Part model, mm, in its own coordinate system. A direction names the side the tool comes from. Round coordinates to 2 decimals unless told otherwise and drop trailing zeros. Loops run counter-clockwise (first coordinate to the right, second up) from the corner with the lowest first, then second, coordinate; pieces in that order, holes last.
from build123d import *

# Parameters (mm, degrees)
SKETCH1_W           = 84
SKETCH1_H           = 300
SKETCH1_W_2         = 54
SKETCH1_H_2         = 80
BOSS_EXTRUDE1_DEPTH = 6
SKETCH2_R           = 1
CUT_EXTRUDE1_DEPTH  = 10
SKETCH4_R           = 1
CUT_EXTRUDE3_DEPTH  = 10
SKETCH5_R           = 1
CUT_EXTRUDE4_DEPTH  = 10


with BuildPart() as part:
    # Sketch1 → Boss-Extrude1 (new body)
    with BuildSketch(Plane.XY):
        Rectangle(SKETCH1_W, SKETCH1_H)
        with Locations((0, 95)):
            Rectangle(SKETCH1_W_2, SKETCH1_H_2, mode=Mode.SUBTRACT)
        with Locations((0, -95)):
            Rectangle(SKETCH1_W_2, SKETCH1_H_2, mode=Mode.SUBTRACT)
        Rectangle(SKETCH1_W_2, SKETCH1_H_2, mode=Mode.SUBTRACT)
    extrude(amount=BOSS_EXTRUDE1_DEPTH)

    # Sketch2 → Cut-Extrude1 (cut)
    with BuildSketch(Plane(origin=(42, 0, 0), x_dir=(0, 0, -1), z_dir=(1, 0, 0))):
        with Locations((-3, 146)):
            Circle(SKETCH2_R)
        with Locations((-3, 0)):
            Circle(SKETCH2_R)
        with Locations((-3, -146)):
            Circle(SKETCH2_R)
        with Locations((-3, -292)):
            Circle(SKETCH2_R)
    cut_extrude1 = extrude(amount=-CUT_EXTRUDE1_DEPTH, mode=Mode.SUBTRACT)

    # Mirror1: Cut-Extrude1 across plane
    add(cut_extrude1.mirror(Plane(origin=(0, 0, 0), x_dir=(0, 0, 1), z_dir=(1, 0, 0))), mode=Mode.SUBTRACT)

    # Sketch4 → Cut-Extrude3 (cut)
    with BuildSketch(Plane.XY.offset(6)):
        with Locations((-14.5, 146.5)):
            Circle(SKETCH4_R)
        with Locations((-33, 122)):
            Circle(SKETCH4_R)
        with Locations((-14.5, 47.5)):
            Circle(SKETCH4_R)
        with Locations((-14.5, -47.5)):
            Circle(SKETCH4_R)
        with Locations((-14.5, -146.5)):
            Circle(SKETCH4_R)
        with Locations((-33, -125)):
            Circle(SKETCH4_R)
        with Locations((-33, 77)):
            Circle(SKETCH4_R)
        with Locations((-33, -80)):
            Circle(SKETCH4_R)
        with Locations((-33, 21)):
            Circle(SKETCH4_R)
        with Locations((-33, -24)):
            Circle(SKETCH4_R)
        with Locations(Location((33, -24, 0), (0, 0, 180))):
            Circle(SKETCH4_R)
        with Locations(Location((33, 21, 0), (0, 0, 180))):
            Circle(SKETCH4_R)
        with Locations(Location((33, -80, 0), (0, 0, 180))):
            Circle(SKETCH4_R)
        with Locations(Location((33, 77, 0), (0, 0, 180))):
            Circle(SKETCH4_R)
        with Locations(Location((33, -125, 0), (0, 0, 180))):
            Circle(SKETCH4_R)
        with Locations(Location((14.5, -146.5, 0), (0, 0, 180))):
            Circle(SKETCH4_R)
        with Locations(Location((14.5, -47.5, 0), (0, 0, 180))):
            Circle(SKETCH4_R)
        with Locations(Location((14.5, 47.5, 0), (0, 0, 180))):
            Circle(SKETCH4_R)
        with Locations(Location((33, 122, 0), (0, 0, 180))):
            Circle(SKETCH4_R)
        with Locations(Location((14.5, 146.5, 0), (0, 0, 180))):
            Circle(SKETCH4_R)
    extrude(amount=-CUT_EXTRUDE3_DEPTH, mode=Mode.SUBTRACT)

    # Sketch5 → Cut-Extrude4 (cut)
    with BuildSketch(Plane.XY.offset(6)):
        with Locations((-37, -143)):
            Circle(SKETCH5_R)
        with Locations((37, -143)):
            Circle(SKETCH5_R)
        with Locations((-37, 143)):
            Circle(SKETCH5_R)
        with Locations((37, 143)):
            Circle(SKETCH5_R)
    extrude(amount=-CUT_EXTRUDE4_DEPTH, mode=Mode.SUBTRACT)


solid = part.part
1) Mould opens along X. For faces 3 (the face through (42, -2, 3)), 4 (the face through (27, 94, 3)), 5 (the face through (-1, 150, 3)) say: released by +X, released by -X, zero draft, split by the parting line, or undercut.
Values:
face 3: released by +X
face 4: undercut
face 5: zero draft
2) Slice it at B-B, the plane y = -99. Give the cut face in (x, z).
Values:
outline: (-42, 0) - (-27, 0) - (-27, 6) - (-42, 6) - close; (27, 0) - (42, 0) - (42, 6) - (27, 6) - close
3) Slice it at C-C, the plane z = 3. Give the number of separate pieces and of enclosed holes in the cut face, then the cut area to 3 significant figures.
Values:
separate pieces: 1
enclosed holes: 27
area: 12,000 mm2
4) Drop flat-ended pins along their axis: pin 1 Ø1.8 at (y, z) = (146, 3) entering from +X; pin 2 Ø0.6 at (y, z) = (-146.5, 3) entering from -X. Give the stop position or say it passes through.
Values:
pin 1: stops at x = 32
pin 2: stops at x = -32
5) Slice it at A-A, the plane x = 5. Give the cut face in (y, z), then the cut area to 3 significant figures.
Values:
outline: (-150, 0) - (-135, 0) - (-135, 6) - (-150, 6) - close; (-55, 0) - (-40, 0) - (-40, 6) - (-55, 6) - close; (40, 0) - (55, 0) - (55, 6) - (40, 6) - close; (135, 0) - (150, 0) - (150, 6) - (135, 6) - close
area: 360 mm2
6) Tool access for faces 1 (the face through (0, 135, 3)), 2 (the face through (-42, -2, 3)): list every direction of +Z, -Z, +X, -X, +Y, -Y with a clear straight run to the whole face (end or side of a thin tool).
Values:
face 1: +Z, -Z
face 2: +Z, -Z, -X, +Y, -Y
7) Wall check: line 1 along Y through (x, z) = (-22, 1.6); line 2 along Y through (x, z) = (37, 1.2); line 3 along X through (y, z) = (77, 2). Give the ranges that are in metal, low to high.
Values:
line 1: y = -150 to -135, -55 to -40, 40 to 55, 135 to 150
line 2: y = -150 to -144, -142 to 142, 144 to 150
line 3: x = -42 to -34, -32 to -27, 27 to 32, 34 to 42
